Autodesk Inventor part; units mm, degrees
ref_plane "YZ Plane" through (0, 0, 0) normal (1, 0, 0) x (0, 1, 0)
ref_plane "XZ Plane" through (0, 0, 0) normal (0, 1, 0) x (-1, 0, 0)
ref_plane "XY Plane" through (0, 0, 0) normal (0, 0, 1) x (1, 0, 0)
sketch "Sketch1" plane through (0, 0, 0) normal (0, 0, 1) x (1, 0, 0)
  line L0 (33.02, -67.31) -> (-33.02, -67.31)
  line L1 (-33.02, -67.31) -> (-33.02, 67.31)
  line L2 (-33.02, 67.31) -> (33.02, 67.31)
  line L3 (33.02, 67.31) -> (33.02, -67.31)
  line L4 (33.02, -67.31) -> (-33.02, 67.31) construction
  line L5 (-33.02, -67.31) -> (33.02, 67.31) construction
  point P0 (0, 0)
  dimension "d0" = 66.04
  dimension "d1" = 134.62
extrude "Extrusion1" add sketch "Sketch1" along normal blind 10.16
fillet "Fillet1" radius 10 4 edges at (33.02, 67.31, 5.08) (-33.02, 67.31, 5.08) (33.02, -67.31, 5.08) (-33.02, -67.31, 5.08)
fillet "Fillet2" radius 4 8 edges at (30.0911, -64.3811, 0) (0, -67.31, 0) (-30.0911, -64.3811, 0) (-33.02, 0, 0) (-30.0911, 64.3811, 0) (0, 67.31, 0) (30.0911, 64.3811, 0) (33.02, 0, 0)
fillet "Fillet3" radius 1 8 edges at (30.0911, 64.3811, 10.16) (0, 67.31, 10.16) (-30.0911, 64.3811, 10.16) (-33.02, 0, 10.16) (-30.0911, -64.3811, 10.16) (0, -67.31, 10.16) (30.0911, -64.3811, 10.16) (33.02, 0, 10.16)
properties part number "Andoid Phone" material "ABS Plastic"
Part model, mm, in its own coordinate system. Round coordinates to 2 decimals unless told otherwise and drop trailing zeros. Order: outer loops, then holes, each group sorted by start corner. A loop starts at its lowest first (then second) coordinate and runs counter-clockwise, first axis right, second up. Notation, with made-up numbers: M 61.25,-16.75 L 71.25,-16.75 A35 cw 71.25,15.25 Z; hole C -14,19 d7. An arc over 180 degrees is marked long. Answer in a Markdown table with one row per item. Add a question column.
Q1. Cut at A-A on z = 2. Give the cut face in (x, y), and give its area (3 significant figures).
Q2. Wall check: L1, parallel to Y at x = 5, z = 2.25; L2, parallel to X at y = -46, z = 9.5; L3, parallel to X at y = -51, z = 3.25. Give the ranges that are in metal, low to high. Write a range as from..to.
Q3. Pin check, flat tip, straight feed: pin 1 (1.5 mm diameter, centred on y = 32.5, z = 3, fed in from +X). Stop position of the tip, or through.
Established:
| question | item | result |
|---|---|---|
| 1 | outline | M -32.48,-57.31 A9.46 ccw -23.02,-66.77 L 23.02,-66.77 A9.46 ccw 32.48,-57.31 L 32.48,57.31 A9.46 ccw 23.02,66.77 L -23.02,66.77 A9.46 ccw -32.48,57.31 Z |
| 1 | area | 8,600 mm2 |
| 2 | L1 | y = -66.91..66.91 |
| 2 | L2 | x = -32.96..32.96 |
| 2 | L3 | x = -32.95..32.95 |
| 3 | pin 1 | stops at x = 33.01 |
